```python
from build123d import *

# Parameters (mm, degrees)
ESQUISSE1_W        = 8
ESQUISSE1_H        = 25
ESQUISSE1_R        = 1.75
BOSS_EXTRU_1_DEPTH = 3
ESQUISSE2_W        = 8
ESQUISSE2_H        = 20
ESQUISSE2_R        = 1.75
BOSS_EXTRU_2_DEPTH = 4
CONG_1_R           = 2


with BuildPart() as part:
    # Esquisse1 → Boss.-Extru.1 (new body)
    with BuildSketch(Plane(origin=(0, 0, 0), x_dir=(1, 0, 0), z_dir=(0, 1, 0))):
        Rectangle(ESQUISSE1_W, ESQUISSE1_H)
        with Locations((0, 9.5)):
            Circle(ESQUISSE1_R, mode=Mode.SUBTRACT)
    extrude(amount=BOSS_EXTRU_1_DEPTH)

    # Esquisse2 → Boss.-Extru.2 (add)
    with BuildSketch(Plane.XY.offset(12.5)):
        with Locations((0, -7)):
            Rectangle(ESQUISSE2_W, ESQUISSE2_H)
        with Locations((0, -14)):
            Circle(ESQUISSE2_R, mode=Mode.SUBTRACT)
    extrude(amount=BOSS_EXTRU_2_DEPTH)

    # Congé1
    cong_1_edges = [part.edges().sort_by_distance(p)[0] for p in [
        (0, 3, 16.5),
        (-4, -17, 14.5),
        (4, -17, 14.5),
        (-4, 1.5, -12.5),
        (4, 1.5, -12.5),
    ]]
    fillet(cong_1_edges, radius=CONG_1_R)


solid = part.part
```
Here's how the part is built. I have some questions about the finished solid (model axes, mm). A direction names the side the tool comes from. Round coordinates to 2 decimals unless told otherwise and drop trailing zeros. Write each loop counter-clockwise with the first axis right and the second up, starting at its lowest first coordinate (ties: lowest second). Pieces come first, ordered by that corner, then holes.
Q1. Will these pins go through, and if not, where does the flat tip stop? P1, Ø2.5, axis at x = 1.5, y = -4.5, coming from the -Z side; P2, Ø4, axis at x = 2.5, z = 4.5, coming from the -Y side; P3, Ø12, axis at y = -9.5, z = -2.5, coming from the +X side.
Q2. If we section it at B-B on z = -9.5: Write out the boundary of the cut face in (x, y), plus the area to 3 significant figures.
Q3. If we section it at D-D on y = -1.5: Write out the boundary of the cut face in (x, z).
Q4. If we mould it in two halves opening along Y, with no side actions, what happens to faces 1 (the cylindrical face through (-0.228, -12.265, 14.472)), 2 (the cylindrical face through (3.43, 1.52, -11.9)), 3 (the flat face through (0, -17, 14)), 4 (the cylindrical face through (0.06, 2.43, 15.9))? For each: +Y half, -Y half, draft (parallel to the pull), parting line (faces both ways), or undercut.
Q5. If we section it at C-C on x = 0: Write out the boundary of the cut face in (y, z), plus the area to 3 significant figures.
Q6. If we section it at A-A on y = -14: Write out the boundary of the cut face in (x, z), plus the area to 3 significant figures.
Q7. Which directions (+Z, -Z, +X, -X, +Y, -Y) give clear straight access to the entire face, cutting with the end or side of a thin tool? Please do faces 5 (the flat face through (0, -8, 12.5)), 6 (the cylindrical face through (3.43, -16.4, 14.53)).
Q8. Please list where these lines run through material, in increasing order: probe 1 along X at (y, z) = (0.65, -9.5); probe 2 along Y at (x, z) = (2.75, -4.25); probe 3 along Z at (x, y) = (0.5, -0.5).
Answer below:
1. P1: stops at z = 12.5
1. P2: stops at y = 0
1. P3: passes through
2. outline: (-4, 0) - (-1.75, 0) - (-1.75, 3) - (-4, 3) - close; (1.75, 0) - (4, 0) - (4, 3) - (1.75, 3) - close
2. area: 13.5 mm2
3. outline: (-4, 12.5) - (4, 12.5) - (4, 16.5) - (-4, 16.5) - close
4. face 1: undercut
4. face 2: draft
4. face 3: -Y half
4. face 4: +Y half
5. outline: (-17, 12.5) - (-15.75, 12.5) - (-15.75, 16.5) - (-17, 16.5) - close; (-12.25, 12.5) - (0, 12.5) - (0, -7.75) - (3, -7.75) - (3, 14.5) arc R2 ccw to (1, 16.5) - (-12.25, 16.5) - close; (0, -12.5) - (3, -12.5) - (3, -11.25) - (0, -11.25) - close
5. area: 130 mm2
6. outline: (-4, 12.5) - (-1.75, 12.5) - (-1.75, 16.5) - (-4, 16.5) - close; (1.75, 12.5) - (4, 12.5) - (4, 16.5) - (1.75, 16.5) - close
6. area: 18.0 mm2
7. face 5: -Z, +X, -X, -Y
7. face 6: +Z, -Z, +X, -Y
8. probe 1: x = -4 to -1.75, 1.75 to 4
8. probe 2: y = 0 to 3
8. probe 3: z = 12.5 to 16.5
